Check sheet for the modelled part. Datum: model origin and axes. Units: mm. Round coordinates to 2 decimals unless told otherwise and drop trailing zeros. Write each loop counter-clockwise with the first axis right and the second up, starting at its lowest first coordinate (ties: lowest second). Pieces come first, ordered by that corner, then holes.
Item 1: Cross-section at C-C on z = -3. Enter the section's corners in (x, y), plus the area to 3 significant figures.
Item 2: Material ranges on line 1 (Z direction, x = -4, y = 278); line 2 (X direction, y = 221, z = -2.25); line 3 (X direction, y = 218, z = -1.25), recorded low to high.
Item 3: Cross-section at B-B on y = 105.5. Enter the section's corners in (x, z).
Item 4: Go/stop test with flat-tipped pins: pin 1 Ø1 at (y, z) = (221, -2) entering from +X; pin 2 Ø2 at (y, z) = (69.5, -3.5) entering from -X. Record where each tip stops, or that it passes through.
Item 5: Cross-section at A-A on x = -1. Enter the section's corners in (y, z), plus the area to 3 significant figures.
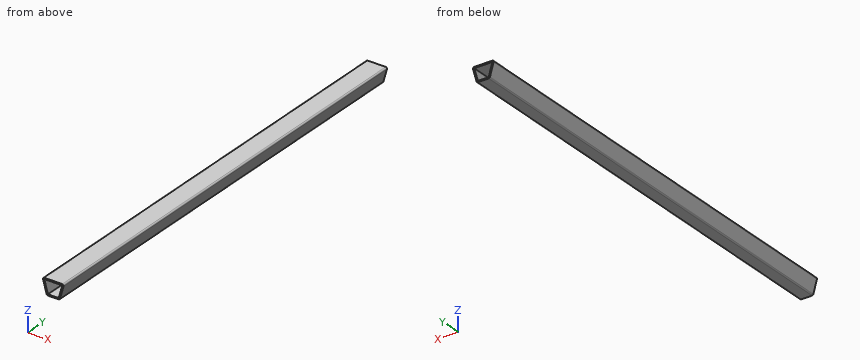
from build123d import *

# Parameters (mm, degrees)
BOSS_EXTRUDE1_DEPTH = 350


with BuildPart() as part:
    # Sketch1 → Boss-Extrude1 (new body)
    with BuildSketch(Plane(origin=(0, 0, 0), x_dir=(1, 0, 0), z_dir=(0, 1, 0))):
        with BuildLine():
            Line((-7.039855599, -6), (7.039855599, -6))
            ThreePointArc((7.039855599, -6), (7.836958346, -5.603843698), (8.002506539, -4.729254423))
            Line((8.002506539, -4.729254423), (5.190006539, 5.270745577))
            ThreePointArc((5.190006539, 5.270745577), (4.831199297, 5.797102746), (4.227355599, 6))
            Line((4.227355599, 6), (-4.227355599, 6))
            ThreePointArc((-4.227355599, 6), (-4.831199297, 5.797102746), (-5.190006539, 5.270745577))
            Line((-5.190006539, 5.270745577), (-8.002506539, -4.729254423))
            ThreePointArc((-8.002506539, -4.729254423), (-7.836958346, -5.603843698), (-7.039855599, -6))
        make_face()
        Polygon((-7.039855599, -5), (7.039855599, -5), (4.227355599, 5), (-4.227355599, 5), align=None, mode=Mode.SUBTRACT)
    extrude(amount=BOSS_EXTRUDE1_DEPTH)


solid = part.part
Response values:
1. outline: (-5.83, 0) - (-4.79, 0) - (-4.79, 350) - (-5.83, 350) - close; (4.79, 0) - (5.83, 0) - (5.83, 350) - (4.79, 350) - close
1. area: 727 mm2
2. line 1: z = -6 to -5, 5 to 6
2. line 2: x = -6.04 to -5, 5 to 6.04
2. line 3: x = -6.32 to -5.28, 5.28 to 6.32
3. outline: (-8, 4.73) - (-5.19, -5.27) arc R1 ccw to (-4.23, -6) - (4.23, -6) arc R1 ccw to (5.19, -5.27) - (8, 4.73) arc R1 ccw to (7.04, 6) - (-7.04, 6) arc R1 ccw to start; hole (-7.04, 5) - (-4.23, -5) - (4.23, -5) - (7.04, 5) - close
4. pin 1: stops at x = 6.25
4. pin 2: stops at x = -5.97
5. outline: (0, -6) - (350, -6) - (350, -5) - (0, -5) - close; (0, 5) - (350, 5) - (350, 6) - (0, 6) - close
5. area: 700 mm2
